Could you check a few things on this model? Use its own coordinates, in mm. Face numbers are marked on the shaded views. A direction names the side the tool comes from. Give positions to 0.01 mm unless a question says otherwise; leave off trailing zeros. Write each loop counter-clockwise with the first axis right and the second up, starting at its lowest first coordinate (ties: lowest second). Pieces come first, ordered by that corner, then holes. Notation, with made-up numbers: M 15.25,42.5 L 69.25,42.5 A29 cw 69.25,70.5 Z; hole C 43,46 d6. An arc over 180 degrees is marked long. Write each question's results on one line, items separated by ' | '. Start each with the question number.
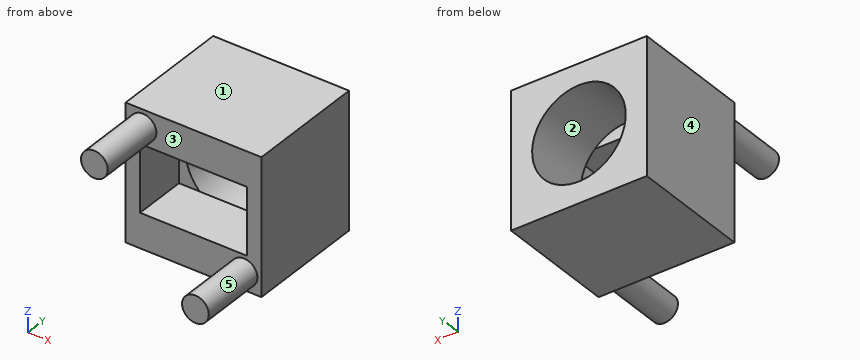
from build123d import *

# Parameters (mm, degrees)
SKETCH1_W           = 5.08
SKETCH1_H           = 5.08
SKETCH1_W_2         = 4
SKETCH1_H_2         = 2.5
BOSS_EXTRUDE1_DEPTH = 2
SKETCH2_W           = 5.08
SKETCH2_H           = 5.08
SKETCH2_R           = 1.75
BOSS_EXTRUDE2_DEPTH = 2.5
SKETCH1_3_R         = 0.5
BOSS_EXTRUDE3_DEPTH = 2.5


with BuildPart() as part:
    # Sketch1 → Boss-Extrude1 (new body)
    with BuildSketch(Plane(origin=(0, 0, 0), x_dir=(1, 0, 0), z_dir=(0, 1, 0))):
        Rectangle(SKETCH1_W, SKETCH1_H)
        Rectangle(SKETCH1_W_2, SKETCH1_H_2, mode=Mode.SUBTRACT)
    extrude(amount=BOSS_EXTRUDE1_DEPTH)

    # Sketch2 → Boss-Extrude2 (add)
    with BuildSketch(Plane(origin=(0, 2, 0), x_dir=(1, 0, 0), z_dir=(0, 1, 0))):
        Rectangle(SKETCH2_W, SKETCH2_H)
        with Locations(Location((0, 0, 0), (0, 0, 45.584691403))):
            Circle(SKETCH2_R, mode=Mode.SUBTRACT)
    extrude(amount=BOSS_EXTRUDE2_DEPTH)

    # Sketch1_3 → Boss-Extrude3 (add)
    with BuildSketch(Plane(origin=(0, 0, 0), x_dir=(1, 0, 0), z_dir=(0, 1, 0))):
        with Locations(Location((-1.89, -1.89, 0), (0, 0, 270))):
            Circle(SKETCH1_3_R)
        with Locations(Location((1.89, 1.89, 0), (0, 0, 270))):
            Circle(SKETCH1_3_R)
    extrude(amount=-BOSS_EXTRUDE3_DEPTH)


solid = part.part
Q1. If we section it at A-A (z = 0): Please give me the cut outline in (x, y).
Q2. Please list where these lines run through material, in increasing order: line 1 (X direction, y = 3.55, z = 0); line 2 (X direction, y = 0.5, z = 0.4). Write a range as [from, to].
Q3. For the marked faces 4 and 5, which set-ups out of +Z, -Z, +X, -X, +Y, -Y let a thin tool reach every point of the face, with its end or its side?
Q4. If we section it at D-D (x = -1.89): Please give me the cut outline in (y, z), plus the area to 3 significant figures.
Q5. I'm going to push flat-ended pins straight in: P1, Ø1.5, axis at x = 0, z = 1, coming from the -Y side; P2, Ø0.6, axis at x = -1.5, z = -0.5, coming from the -Y side. Where does each tip first touch, or does it pass through?
Q6. If we section it at C-C (x = -0.75): Please give me the cut outline in (y, z).
Q7. If we mould it in two halves opening along Z, with no side actions, what happens to the marked faces 1, 2 and 3? For each: pulls with the +Z half, pulls with the -Z half, needs draft (parallel to the pull), parting line crosses it, or undercut.
Q8. If we section it at B-B (y = 2.25): Please give me the cut outline in (x, z).
Determined:
1) outline: M -2.54,0 L -2,0 L -2,2 L -1.75,2 L -1.75,4.5 L -2.54,4.5 Z; M 1.75,2 L 2,2 L 2,0 L 2.54,0 L 2.54,4.5 L 1.75,4.5 Z
2) line 1: x = [-2.54, -1.75], [1.75, 2.54] | line 2: x = [-2.54, -2], [2, 2.54]
3) face 4: +Z, -Z, -X, +Y, -Y | face 5: -Y
4) outline: M -2.5,1.39 L 0,1.39 L 0,1.25 L 2,1.25 L 2,-1.25 L 0,-1.25 L 0,-2.54 L 4.5,-2.54 L 4.5,2.54 L 0,2.54 L 0,2.39 L -2.5,2.39 Z | area: 20.4 mm²
5) P1: stops at y = 0 | P2: stops at y = 2
6) outline: M 0,-2.54 L 4.5,-2.54 L 4.5,-1.58 L 2,-1.58 L 2,-1.25 L 0,-1.25 Z; M 0,1.25 L 2,1.25 L 2,1.58 L 4.5,1.58 L 4.5,2.54 L 0,2.54 Z
7) face 1: pulls with the +Z half | face 2: undercut | face 3: needs draft
8) outline: M -2.54,-2.54 L 2.54,-2.54 L 2.54,2.54 L -2.54,2.54 Z; hole C 0,0 d3.5
